from build123d import *

# Parameters (mm, degrees)
SKETCH_1_W                       = 158
SKETCH_1_H                       = 125
SM_BASE_FLANGE_1_DEPTH           = 2
SM_EDGE_FLANGE_1_STRIP_W         = 9.4732
SM_EDGE_FLANGE_1_STRIP_H         = 2
SM_EDGE_FLANGE_1_STRIP_CUT_DEPTH = 158
SM_EDGE_FLANGE_1_DEPTH           = 158
SM_BASE_FLANGE_1_2_DEPTH         = 2


# Sheet-metal steps are written as plain solids
with BuildPart() as part:
    # Sketch 1 → Sm Base Flange 1 (new body)
    with BuildSketch(Plane(origin=(0, 0, 0), x_dir=(1, 0, 0), z_dir=(0, 1, 0))):
        Rectangle(SKETCH_1_W, SKETCH_1_H)
    extrude(amount=-SM_BASE_FLANGE_1_DEPTH)

    # 边线-法兰1 strip (across the edge) → 边线-法兰1 strip cut (cut)
    with BuildSketch(Plane(origin=(79, -2, 62.5), x_dir=(0, 0, -1), z_dir=(-1, 0, 0))):
        with Locations((-2, -1)):
            Rectangle(SM_EDGE_FLANGE_1_STRIP_W, SM_EDGE_FLANGE_1_STRIP_H)
    extrude(amount=SM_EDGE_FLANGE_1_STRIP_CUT_DEPTH, mode=Mode.SUBTRACT)

    # 边线-法兰1 section (across the edge) → 边线-法兰1 (add)
    with BuildSketch(Plane(origin=(79, -2, 62.5), x_dir=(0, 0, -1), z_dir=(-1, 0, 0))):
        with BuildLine():
            Line((0, 0.7366), (0, 67))
            Line((0, 67), (2, 67))
            Line((2, 67), (2, 0.7366))
            ThreePointArc((2, 0.7366), (2.215745145, 0.215745145), (2.7366, 0))
            Line((2.7366, 0), (2.7366, -2))
            ThreePointArc((2.7366, -2), (0.801531583, -1.198468417), (0, 0.7366))
        make_face()
    extrude(amount=SM_EDGE_FLANGE_1_DEPTH)

    # 草图9 → Sm Base Flange 1 2 (add)
    with BuildSketch(Plane.XY.offset(62.5)):
        Polygon((-79, -2.7366), (-108.732309369, -56), (-108.732309369, -69), (110.643827525, -69), (110.643827525, -44), (79, -2.7366), align=None)
    extrude(amount=-SM_BASE_FLANGE_1_2_DEPTH)


solid = part.part
Geometry: final body of the model. Coordinates: model frame, mm. A direction names the side the tool comes from. Round coordinates to 2 decimals unless told otherwise and drop trailing zeros. Loops run counter-clockwise (first coordinate to the right, second up) from the corner with the lowest first, then second, coordinate; pieces in that order, holes last.
Q1. Access query for faces 1 (the flat face through (-93.66, -29, 61.51)), 2 (the flat face through (-1, -2, -2)). Directions: +Z, -Z, +X, -X, +Y, -Y. A direction counts if a zero-diameter tool reaches every point of the face in a straight line with its end or side. Return the directions, or none.
Q2. Pin query (flat end, axial travel): P1, Ø8, axis at x = 47, y = -24, coming from the -Z side; P2, Ø5, axis at x = -3.5, z = -9.5, coming from the -Y side; P3, Ø1.4, axis at y = -1.5, z = 0.5, coming from the -X side. Return the tip coordinate at first contact, or that it passes through.
Q3. Section A-A on x = 66.5. Return loops of the section in (y, z), plus the area to 3 significant figures.
Q4. Section C-C on y = -62.5. Return loops of the section in (x, z).
Q5. Section B-B on z = 33.5. Return loops of the section in (x, y), plus the area to 3 significant figures.
Q6. Material intervals for L1, parallel to Y at x = -16, z = -47; L2, parallel to Z at x = -8, y = -58, sorted ascending.
Evaluation:
1. face 1: +Z, -Z, -X, +Y
1. face 2: -Z, +X, -X, -Y
2. P1: stops at z = 60.5
2. P2: stops at y = -2
2. P3: stops at x = -79
3. outline: (-69, 60.5) - (-2.74, 60.5) arc R0.74 cw to (-2, 59.76) - (-2, -62.5) - (0, -62.5) - (0, 59.76) arc R2.74 ccw to (-2.74, 62.5) - (-69, 62.5) - close
3. area: 383 mm2
4. outline: (-108.73, 60.5) - (110.64, 60.5) - (110.64, 62.5) - (-108.73, 62.5) - close
5. outline: (-79, -2) - (79, -2) - (79, 0) - (-79, 0) - close
5. area: 316 mm2
6. L1: y = -2 to 0
6. L2: z = 60.5 to 62.5
